Source: CAD feature listing. Evaluate the final solid. Frame: model axes, mm. Face numbers are marked on the shaded views. A direction names the side the tool comes from. Give positions to 0.01 mm unless a question says otherwise; leave off trailing zeros. Write each loop counter-clockwise with the first axis right and the second up, starting at its lowest first coordinate (ties: lowest second). Pieces come first, ordered by that corner, then holes. Notation, with made-up numbers: (-10, 4.25) -> (7, 4.25) arc R12 ccw to (7, 26.25) -> close; hole circle Ø2 at (-0.5, -31). An arc over 180 degrees is marked (long way). Answer as a JSON object with one key per item and string values. Group by question number.
Item 1: Ray query, probe 1 along X at (y, z) = (147.5, -253); probe 2 along X at (y, z) = (45.5, -256); probe 3 along Z at (x, y) = (47, 226.5). Return the intervals inside material, ascending. Write a range as from..to.
Item 2: Access query for the marked faces 5 and 6. Directions: +Z, -Z, +X, -X, +Y, -Y. A direction counts if a zero-diameter tool reaches every point of the face in a straight line with its end or side. Return the directions, or none.
Item 3: Pull-direction query (X, two-part tool) for the marked faces 1, 2, 3 and 4; classes: pulls with the +X half, pulls with the -X half, needs draft (parallel to the pull), parting line crosses it, or undercut.
Item 4: Section query A-A on x = 129. Return the cut outline in (y, z).
Item 5: First-contact query: pin 1 Ø8 at (y, z) = (-379.5, -170) entering from -X; pin 2 Ø3 at (x, y) = (130.5, 306.5) entering from -Z; pin 3 Ø5 at (x, y) = (81, -377.5) entering from -Z; pin 4 Ø1 at (y, z) = (345.5, -201.5) entering from +X. Flat tips, straight axial feed; report the tip coordinate or a pass-through.
Item 6: Section query B-B on y = -141. Return the cut outline in (x, z).
Item 7: Section query C-C on z = -274.5. Return the cut outline in (x, y), plus the area to 3 significant figures.
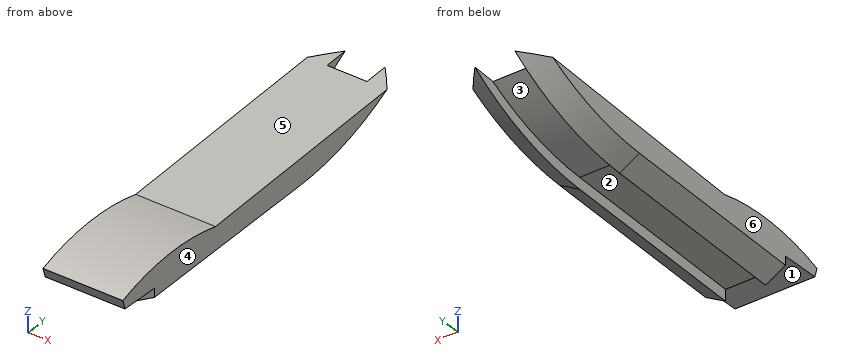
from build123d import *

# Parameters (mm, degrees)
F1_DEPTH = 254
F5_DEPTH = 307.34


with BuildPart() as f1:
    # F0 (on Right) → F1 (new body)
    with BuildSketch(Plane.YZ):
        with BuildLine():
            ThreePointArc((124.7064843774, -223.4433591366), (347.4699832399, -182.0563968003), (550.3501296043, -81.1797231436))
            Line((550.3501296043, -81.1797231436), (-238.9836609364, -132.8076571226))
            ThreePointArc((-238.9836609364, -132.8076571226), (-435.8096530096, -129.9809624391), (-625.6195306778, -182.1410208941))
            Line((-625.6195306778, -182.1410208941), (-612.9993796349, -223.4433591366))
            Line((-612.9993796349, -223.4433591366), (-489.0923500061, -223.4433591366))
            Line((-489.0923500061, -223.4433591366), (-489.0923500061, -250.9782612324))
            Line((-489.0923500061, -250.9782612324), (124.7064843774, -223.4433591366))
        make_face()
    extrude(amount=F1_DEPTH)

    # F3: sweep along a path in F3_path
    with BuildLine(Plane(origin=(0, 124.7064843774, -223.4433591366), x_dir=(0, 0, -1), z_dir=(-1, 0, 0))) as f3_path:
        Line((27.5349020958, 613.7988343835), (0, 0))
        ThreePointArc((0, 0), (-41.3869623363, -222.7634988625), (-142.263635993, -425.643645227))
    # F2 (on face) → F3 (sweep)
    with BuildSketch(Plane.XZ.offset(489.0923500061)):
        Polygon((63.5, -286.5382612324), (63.5, -250.9782612324), (0, -250.9782612324), align=None)
        Polygon((254, -250.9782612324), (190.5, -250.9782612324), (190.5, -286.5382612324), align=None)
    sweep(path=f3_path.line)

    # F4 (on face) → F5 (cut)
    with BuildSketch(Plane(origin=(0, 0, 0), x_dir=(0, -1, 0), z_dir=(-1, 0, 0))):
        with BuildLine():
            Line((622.0669402345, -193.7676877722), (640.6544446945, -195.0154304504))
            Line((640.6544446945, -195.0154304504), (549.1129755974, -11.9324130937))
            Line((549.1129755974, -11.9324130937), (-511.2428665161, 10.9529634938))
            Line((-511.2428665161, 10.9529634938), (-584.1369628906, -112.79758811))
            Line((-584.1369628906, -112.79758811), (232.107648548, -167.5904861977))
            ThreePointArc((232.107648548, -167.5904861977), (429.0143567126, -151.9718221639), (622.0669402345, -193.7676877722))
        make_face()
    extrude(amount=-F5_DEPTH, mode=Mode.SUBTRACT)


solid = f1.part
Worked answers:
{
 "1": {"probe 1": "55.09..63.5, 190.5..198.91", "probe 2": "51.79..63.5, 190.5..202.21", "probe 3": "-239.13..-136.81"},
 "2": {"face 5": "+Z, +X, -X", "face 6": "+Z, -Z, -X, +Y, -Y"},
 "3": {"face 1": "needs draft", "face 2": "undercut", "face 3": "undercut", "face 4": "pulls with the +X half"},
 "4": {"outline": "(-622.07, -193.77) -> (-613, -223.44) -> (-489.09, -223.44) -> (-489.09, -250.98) -> (124.71, -223.44) arc R818.44 ccw to (489.26, -119.17) -> (-232.11, -167.59) arc R678.03 ccw to start"},
 "5": {"pin 1": "x = 0", "pin 2": "z = -194.98", "pin 3": "z = -246.08", "pin 4": "x = 222.98"},
 "6": {"outline": "(0, -235.36) -> (63.5, -270.92) -> (63.5, -235.36) -> (190.5, -235.36) -> (190.5, -270.92) -> (254, -235.36) -> (254, -161.47) -> (0, -161.47) -> close"},
 "7": {"outline": "(42, -489.09) -> (63.5, -489.09) -> (63.5, -220.74) -> close; (190.5, -489.09) -> (212, -489.09) -> (190.5, -220.74) -> close", "area": "5,770 mm^2"}
}
